Work out the finished part from the listing and answer in its coordinate system (mm). A direction names the side the tool comes from. Round coordinates to 2 decimals unless told otherwise and drop trailing zeros. Loops run counter-clockwise (first coordinate to the right, second up) from the corner with the lowest first, then second, coordinate; pieces in that order, holes last. Notation, with made-up numbers: (-38.5, 10) - (-20.5, 10) arc R24 ccw to (-20.5, 35) - close; hole circle Ø4 at (4, 11). An arc over 180 degrees is marked (long way). Return JSON: item names as keys, results as strings.
from build123d import *

# Parameters (mm, degrees)
SKETCH2_W           = 6.35
SKETCH2_H           = 5.08
SKETCH2_R           = 1.7
SKETCH2_R_2         = 2.5527
SKETCH2_R_3         = 1
SKETCH2_R_4         = 6.275
BOSS_EXTRUDE1_DEPTH = 5.08
FILLET1_R           = 6.35
FILLET2_R           = 3.175


with BuildPart() as part:
    # Sketch2 → Boss-Extrude1 (new body)
    with BuildSketch(Plane.XY):
        Polygon((-110.49, 12.7), (-120.65, 12.7), (-120.65, -12.7), (-110.49, -12.7), (-110.49, -6.35), (-105.41, -6.35), (-105.41, -12.7), (-78.74, -12.7), (-78.74, -6.35), (-73.66, -6.35), (-73.66, -12.7), (-65.0875, -12.7), (-65.0875, -14.2875), (-61.9125, -14.2875), (-61.9125, -12.7), (87.3125, -12.7), (87.3125, -14.2875), (90.4875, -14.2875), (90.4875, -12.7), (104.775, -12.7), (104.775, -20.9775), (111.125, -20.9775), (111.125, -12.7), (120.65, -12.7), (120.65, 12.7), (111.125, 12.7), (111.125, 20.9775), (104.775, 20.9775), (104.775, 12.7), (90.4875, 12.7), (90.4875, 14.2875), (87.3125, 14.2875), (87.3125, 12.7), (-61.9125, 12.7), (-61.9125, 14.2875), (-65.0875, 14.2875), (-65.0875, 12.7), (-73.66, 12.7), (-73.66, 6.35), (-78.74, 6.35), (-78.74, 12.7), (-105.41, 12.7), (-105.41, 6.35), (-110.49, 6.35), align=None)
        with Locations((-92.075, -8.09625)):
            Rectangle(SKETCH2_W, SKETCH2_H, mode=Mode.SUBTRACT)
        with Locations((-63.5, -9.525)):
            Circle(SKETCH2_R, mode=Mode.SUBTRACT)
        with BuildLine():
            ThreePointArc((-101.6, -3.175), (-104.775, 0), (-101.6, 3.175))
            Line((-101.6, 3.175), (-82.55, 3.175))
            ThreePointArc((-82.55, 3.175), (-79.375, 0), (-82.55, -3.175))
            Line((-82.55, -3.175), (-101.6, -3.175))
        make_face(mode=Mode.SUBTRACT)
        with Locations((-38.1, 0)):
            Circle(SKETCH2_R_2, mode=Mode.SUBTRACT)
        with Locations((-12.7, 0)):
            Circle(SKETCH2_R_2, mode=Mode.SUBTRACT)
        with Locations((107.95, -16.215)):
            Circle(SKETCH2_R_3, mode=Mode.SUBTRACT)
        with Locations((12.7, 0)):
            Circle(SKETCH2_R_2, mode=Mode.SUBTRACT)
        with Locations((38.1, 0)):
            Circle(SKETCH2_R_2, mode=Mode.SUBTRACT)
        with Locations((88.9, -9.525)):
            Circle(SKETCH2_R, mode=Mode.SUBTRACT)
        with Locations((63.5, 0)):
            Circle(SKETCH2_R_2, mode=Mode.SUBTRACT)
        with Locations((107.95, 0)):
            Circle(SKETCH2_R_4, mode=Mode.SUBTRACT)
        with Locations((-92.075, 8.09625)):
            Rectangle(SKETCH2_W, SKETCH2_H, mode=Mode.SUBTRACT)
        with Locations((-63.5, 9.525)):
            Circle(SKETCH2_R, mode=Mode.SUBTRACT)
        with Locations((88.9, 9.525)):
            Circle(SKETCH2_R, mode=Mode.SUBTRACT)
        with Locations((107.95, 16.215)):
            Circle(SKETCH2_R_3, mode=Mode.SUBTRACT)
    extrude(amount=BOSS_EXTRUDE1_DEPTH)

    # Fillet1
    fillet1_edges = [part.edges().sort_by_distance(p)[0] for p in [
        (104.775, 12.7, 2.54),
        (120.65, 12.7, 2.54),
        (120.65, -12.7, 2.54),
        (104.775, -12.7, 2.54),
        (-120.65, -12.7, 2.54),
        (-120.65, 12.7, 2.54),
    ]]
    fillet(fillet1_edges, radius=FILLET1_R)

    # Fillet2
    fillet2_edges = [part.edges().sort_by_distance(p)[0] for p in [
        (104.775, -20.9775, 2.54),
        (111.125, -20.9775, 2.54),
        (111.125, -12.7, 2.54),
        (111.125, 12.7, 2.54),
        (111.125, 20.9775, 2.54),
        (104.775, 20.9775, 2.54),
    ]]
    fillet(fillet2_edges, radius=FILLET2_R - 0.0001)  # a hair under: the kernel refuses the full size


solid = part.part
1) Flat-ended cylindrical pins translate along their axes: pin 1 (1.5 mm diameter, centred on x = -93, z = 3, fed in from -Y); pin 2 (3 mm diameter, centred on x = -112, z = 2, fed in from +Y); pin 3 (2.5 mm diameter, centred on x = -108, z = 3, fed in from -Y). Find the tip coordinate at first contact, or state that the pin passes through.
Verdict:
{"pin 1": "stops at y = -12.7", "pin 2": "stops at y = 12.7", "pin 3": "stops at y = -6.35"}
2) Find the intervals of material crossed by L1, parallel to Y at x = 88.9, z = 2.8 (1 decimal); L2, parallel to Y at x = 107.95, z = 1.35 (1 decimal); L3, parallel to X at y = -6.5, z = 4.5, in increasing order.
Verdict:
{"L1": "y = -14.3 to -11.2, -7.8 to 7.8, 11.2 to 14.3", "L2": "y = -21 to -17.2, -15.2 to -6.3, 6.3 to 15.2, 17.2 to 21", "L3": "x = -120.65 to -110.49, -105.41 to -95.25, -88.9 to -78.74, -73.66 to 120.65"}
3) Section C-C (x = 53) is taken. Give the vertices of the cut face in (y, z), and give its area (3 significant figures).
Verdict:
{"outline": "(-12.7, 0) - (12.7, 0) - (12.7, 5.08) - (-12.7, 5.08) - close", "area": "129 mm2"}
4) A tool of negligible diameter and unlimited length cuts with its end or side. For faces 1 (the flat face through (-112, -12.7, 3)), 2 (the flat face through (-108, 6.35, 3)), 3 (the flat face through (-92, 10.636, 3)), from which of +Z, -Z, +X, -X, +Y, -Y can it reach the whole face along a straight path? Write none if from no direction.
Verdict:
{"face 1": "+Z, -Z, -X, -Y", "face 2": "+Z, -Z, +Y", "face 3": "+Z, -Z"}
5) Determine the mould class of faces 4 (the flat face through (-78.74, -10, 3)), 5 (the flat face through (95, 12.7, 3)), 6 (the cylindrical face through (-10.265, 0.767, 2.504)) for opening direction Y: pulls with the +Y half, pulls with the -Y half, needs draft (parallel to the pull), parting line crosses it, or undercut.
Verdict:
{"face 4": "needs draft", "face 5": "pulls with the +Y half", "face 6": "undercut"}
6) Section B-B (y = 0) is taken. Count the separate pieces of the cut face and the enclosed holes in it, and give its area (3 significant figures).
Verdict:
{"separate pieces": "8", "enclosed holes": "0", "area": "903 mm2"}
7) Section A-A (x = -12.7) is taken. Give the vertices of the cut face in (y, z), and give its area (3 significant figures).
Verdict:
{"outline": "(-12.7, 0) - (-2.55, 0) - (-2.55, 5.08) - (-12.7, 5.08) - close; (2.55, 0) - (12.7, 0) - (12.7, 5.08) - (2.55, 5.08) - close", "area": "103 mm2"}
